The listing builds one solid part. Answer for the finished solid, in the listing's coordinates (mm). Round coordinates to 2 decimals unless told otherwise and drop trailing zeros. One line per item, written item: value. Start each with the question number.
1. For a pull along X with two mould halves and no side action, classify faces 1 (the flat face through (-5, 0, 45)), 2 (the flat face through (2.075, 4.752, 22.185)) as released by +X, released by -X, zero draft, split by the parting line, or undercut.
2. Flat-ended cylindrical pins translate along their axes: P1, Ø2, axis at x = -5, z = 13, coming from the +Y side; P2, Ø1, axis at y = -3, z = 16.5, coming from the +X side; P3, Ø4, axis at x = -4.5, z = 21.5, coming from the -Y side. Find the tip coordinate at first contact, or state that the pin passes through.
3. Straight lines are drawn through the part: line 1 (X direction, y = 0, z = 3); line 2 (Y direction, x = 3.75, z = 21); line 3 (X direction, y = 5, z = 30.5). For each, find the intervals that lie inside material, in ascending order.
from build123d import *

# Parameters (mm, degrees)
PAD_DEPTH    = 45
PAD001_DEPTH = 45


with BuildPart() as mirrored:
    # Sketch → Pad (new body)
    with BuildSketch(Plane(origin=(0, 0, 0), x_dir=(0, 1, 0), z_dir=(0, 0, 1))):
        with BuildLine():
            ThreePointArc((0, 7.6), (-5.374012, 5.374012), (-7.6, 0))
            Line((-7.6, 0), (-4.2, 0))
            ThreePointArc((-4.170238, 0.499113), (-4.192553, 0.25), (-4.2, 0))
            Line((-5.982338, 1.345455), (-4.170238, 0.499113))
            Line((-5.670983, 2.504359), (-5.982338, 1.345455))
            Line((-3.858883, 1.658017), (-5.670983, 2.504359))
            ThreePointArc((-3.357546, 2.523269), (-3.634058, 2.105617), (-3.858883, 1.658017))
            Line((-4.690785, 4.014065), (-3.357546, 2.523269))
            Line((-3.840203, 4.860534), (-4.690785, 4.014065))
            Line((-2.506963, 3.369738), (-3.840203, 4.860534))
            ThreePointArc((-1.639291, 3.866875), (-2.087976, 3.644222), (-2.506963, 3.369738))
            Line((-2.281588, 5.760933), (-1.639291, 3.866875))
            Line((-1.14141, 6.064296), (-2.281588, 5.760933))
            Line((-0.499113, 4.170238), (-1.14141, 6.064296))
            ThreePointArc((0, 4.2), (-0.25, 4.192553), (-0.499113, 4.170238))
            Line((0, 4.2), (0, 7.6))
        make_face()
    pad = extrude(amount=PAD_DEPTH)

    # Mirrored: Pad across Sketch H_Axis
    add(pad.mirror(Plane.ZY))


with BuildPart() as fusion:
    # Sketch001 → Pad001 (new body)
    with BuildSketch(Plane(origin=(0, 0, 0), x_dir=(0, -1, 0), z_dir=(0, 0, 1))):
        with BuildLine():
            ThreePointArc((0, 7.6), (-5.374012, 5.374012), (-7.6, 0))
            Line((-7.6, 0), (-4.2, 0))
            ThreePointArc((-4.170238, 0.499113), (-4.192553, 0.25), (-4.2, 0))
            Line((-5.982338, 1.345455), (-4.170238, 0.499113))
            Line((-5.670983, 2.504359), (-5.982338, 1.345455))
            Line((-3.858883, 1.658017), (-5.670983, 2.504359))
            ThreePointArc((-3.357546, 2.523269), (-3.634058, 2.105617), (-3.858883, 1.658017))
            Line((-4.690785, 4.014065), (-3.357546, 2.523269))
            Line((-3.840203, 4.860534), (-4.690785, 4.014065))
            Line((-2.506963, 3.369738), (-3.840203, 4.860534))
            ThreePointArc((-1.639291, 3.866875), (-2.087976, 3.644222), (-2.506963, 3.369738))
            Line((-2.281588, 5.760933), (-1.639291, 3.866875))
            Line((-1.14141, 6.064296), (-2.281588, 5.760933))
            Line((-0.499113, 4.170238), (-1.14141, 6.064296))
            ThreePointArc((0, 4.2), (-0.25, 4.192553), (-0.499113, 4.170238))
            Line((0, 4.2), (0, 7.6))
        make_face()
    pad001 = extrude(amount=PAD001_DEPTH)

    # Mirrored001: Pad001 across Sketch001 H_Axis
    add(pad001.mirror(Plane(origin=(0, 0, 0), x_dir=(0, 0, 1), z_dir=(1, 0, 0))))

    # Fusion: union Mirrored
    add(mirrored.part)


solid = fusion.part
Answer list:
1. face 1: zero draft
1. face 2: undercut
2. P1: stops at y = 6.46
2. P2: stops at x = 7.18
2. P3: stops at y = -7.18
3. line 1: x = -7.6 to -4.2, 4.2 to 7.6
3. line 2: y = -6.61 to -4.45, -2.85 to -1.89, 1.89 to 2.85, 4.45 to 6.61
3. line 3: x = -5.72 to -2.19, -0.89 to 0.89, 2.19 to 5.72
